from build123d import *

# Parameters (mm, degrees)
F0_W     = 22
F0_H     = 12
F1_DEPTH = 5
F2_W     = 7
F2_H     = 12
F3_DEPTH = 1.5
F5_D     = 3.3


with BuildPart() as f1:
    # F0 (on Top) → F1 (new body)
    with BuildSketch(Plane.XY):
        with Locations((-1.241267357, 2.5510253936)):
            Rectangle(F0_W, F0_H)
    extrude(amount=F1_DEPTH)

    # F2 (on face) → F3 (join)
    with BuildSketch(Plane.XY.offset(5)):
        with Locations((-8.741267357, 2.5510253936)):
            Rectangle(F2_W, F2_H)
    extrude(amount=F3_DEPTH)

    # F5 (through all)
    with Locations(Plane.XY.offset(5)):
        with Locations((-1.241267357, 4.5510253936), (6.758732643, 4.5510253936)):
            Hole(F5_D / 2)


solid = f1.part
Check sheet for the modelled part. Datum: model origin and axes. Units: mm. A direction names the side the tool comes from. Round coordinates to 2 decimals unless told otherwise and drop trailing zeros. Loops run counter-clockwise (first coordinate to the right, second up) from the corner with the lowest first, then second, coordinate; pieces in that order, holes last. Notation, with made-up numbers: M 13,18.5 L 22,18.5 A12 ccw 22,40.5 Z; hole C -24.75,-4.75 d6. An arc over 180 degrees is marked long. One line per question, with ' | ' between items. Start each with the question number.
Item 1: Gauge pin test, flat ends, axial feed: pin 1 Ø3 at (x, y) = (2.5, 5.5) entering from +Z; pin 2 Ø1.2 at (y, z) = (0, 6) entering from +X. Record the tip position at first contact, or that the pin passes through.
Item 2: Section check D-D (y = 5.5). Record the boundary of the cut face in (x, z).
Item 3: Scan lines: probe 1 along X at (y, z) = (4.5, 2); probe 2 along X at (y, z) = (4, 3); probe 3 along Z at (x, y) = (-3.25, 0). Record each from-to range of solid material in increasing order.
Item 4: Set-up check for faces 1 (the face through (-1.4, 2.6, 0)), 2 (the face through (2, 3, 5)): record each of +Z, -Z, +X, -X, +Y, -Y from which the full face is reachable in a straight line by a thin tool's end or side.
Item 5: Section check C-C (z = 5.75). Record the boundary of the cut face in (x, y).
Item 6: Section check A-A (x = -0.5). Record the boundary of the cut face in (y, z).
Item 7: Section check B-B (y = -2). Record the boundary of the cut face in (x, z), and give its area (4 significant figures).
Item 8: Release check for a two-part mould opening along X. For faces 3 (the face through (-1, -3.449, 2)), 4 (the face through (-0.88, 2.94, 2.46)), 5 (the face through (9.759, 2, 2)), 6 (the face through (8.07, 3.55, 2.46)) record: released by +X, released by -X, zero draft, split by the parting line, or undercut.
Worked out:
1) pin 1: z = 5 | pin 2: x = -5.24
2) outline: M -12.24,0 L -2.59,0 L -2.59,5 L -5.24,5 L -5.24,6.5 L -12.24,6.5 Z; M 0.11,0 L 5.41,0 L 5.41,5 L 0.11,5 Z; M 8.11,0 L 9.76,0 L 9.76,5 L 8.11,5 Z
3) probe 1: -12.24 to -2.89, 0.41 to 5.11, 8.41 to 9.76 | probe 2: -12.24 to -2.8, 0.31 to 5.2, 8.31 to 9.76 | probe 3: 0 to 5
4) face 1: -Z, +X, -X, +Y, -Y | face 2: +Z, +X, +Y, -Y
5) outline: M -12.24,-3.45 L -5.24,-3.45 L -5.24,8.55 L -12.24,8.55 Z
6) outline: M -3.45,0 L 3.08,0 L 3.08,5 L -3.45,5 Z; M 6.03,0 L 8.55,0 L 8.55,5 L 6.03,5 Z
7) outline: M -12.24,0 L 9.76,0 L 9.76,5 L -5.24,5 L -5.24,6.5 L -12.24,6.5 Z | area: 120.5 mm^2
8) face 3: zero draft | face 4: undercut | face 5: released by +X | face 6: undercut
